Source: CAD feature listing. Evaluate the final solid. Frame: model axes, mm. Face numbers are marked on the shaded views. A direction names the side the tool comes from. Coordinates: 2 decimals unless noted, no trailing zeros. Order: outer loops, then holes, each group sorted by start corner. A loop starts at its lowest first (then second) coordinate and runs counter-clockwise, first axis right, second up. Notation, with made-up numbers: (47, -21.75) -> (61, -21.75) arc R9 ccw to (61, -8.75) -> close; hole circle Ø6 at (-30, 11.5). An arc over 180 degrees is marked (long way). Write item = value, one per line. Start each with the question number.
Item 1: Section query C-C (z = -56). Output: boundary loops of the cut face in (x, y), then the cut area to 3 significant figures.
Item 2: Mould query, pull axis X, two halves, no side actions, for the marked faces 1, 2 and 3. Classes: released by +X, released by -X, zero draft, split by the parting line, or undercut.
Item 3: Set-up query: the marked faces 4, 5, 6 and 7. Return all of +Z, -Z, +X, -X, +Y, -Y with unobstructed straight access to the full face (end or side cutting, diameter ignored); none if empty.
Item 4: Section query D-D (y = 31). Output: boundary loops of the cut face in (x, z), then the cut area to 3 significant figures.
Item 5: Ray query, line 1 along Z through (x, y) = (42.5, 44.5); line 2 along Z through (x, y) = (38, -8.5); line 3 along Z through (x, y) = (-79, 44.5). Return the intervals inside material, ascending. Write a range as [from, to].
Item 6: Section query B-B (y = 0). Output: boundary loops of the cut face in (x, z), then the cut area to 3 significant figures.
Item 7: Contact query for flat-ended pins moving along their axis: pin 1 (6 mm diameter, centred on y = -36.5, z = -48, fed in from -X); pin 2 (10 mm diameter, centred on x = 25.5, z = 32.5, fed in from -Y); pin 3 (6 mm diameter, centred on y = 2, z = 14, fed in from +X). Output: stop coordinate, or through.
Item 8: Section query A-A (x = 0). Output: boundary loops of the cut face in (y, z), then the cut area to 3 significant figures.
```python
from build123d import *

# Parameters (mm, degrees)
BOSS_EXTRUDE1_DEPTH = 200
BOSS_EXTRUDE2_DEPTH = 5
SKETCH3_R           = 37.5
BOSS_EXTRUDE3_DEPTH = 27
SKETCH4_R           = 37.5
BOSS_EXTRUDE4_DEPTH = 25
SKETCH5_R           = 45
BOSS_EXTRUDE5_DEPTH = 19


with BuildPart() as part:
    # Sketch1 → Boss-Extrude1 (new body)
    with BuildSketch(Plane.XY):
        Polygon((-127.5, 50), (-137.5, -50), (137.5, -50), (127.5, 50), align=None)
    extrude(amount=-BOSS_EXTRUDE1_DEPTH)

    # Sketch2 → Boss-Extrude2 (add)
    with BuildSketch(Plane(origin=(0, 0, 0), x_dir=(-1, 0, 0), z_dir=(0, 0, -1))):
        Polygon((-75, 50), (-65, -50), (65, -50), (75, 50), align=None)
    extrude(amount=-BOSS_EXTRUDE2_DEPTH)

    # Sketch3 → Boss-Extrude3 (add)
    with BuildSketch(Plane.XY.offset(5)):
        Circle(SKETCH3_R)
    extrude(amount=BOSS_EXTRUDE3_DEPTH)

    # Sketch4 → Boss-Extrude4 (add)
    with BuildSketch(Plane.XY.offset(32)):
        with BuildLine():
            ThreePointArc((-13.263603946, -35.076014745), (-37.5, 0), (-13.263603946, 35.076014745))
            Line((-13.263603946, 35.076014745), (-53.023534566, 50))
            Line((-53.023534566, 50), (-77.5, 36.492065403))
            Line((-77.5, 36.492065403), (-70.015632516, -50))
            Line((-70.015632516, -50), (-47.291260559, -50))
            Line((-47.291260559, -50), (-13.263603946, -35.076014745))
        make_face()
        Circle(SKETCH4_R)
        with BuildLine():
            Line((53.023534566, 50), (13.263603946, 35.076014745))
            ThreePointArc((13.263603946, 35.076014745), (30.851540869, 21.317420717), (37.5, 0))
            ThreePointArc((37.5, 0), (30.851540869, -21.317420717), (13.263603946, -35.076014745))
            Line((13.263603946, -35.076014745), (47.291260559, -50))
            Line((47.291260559, -50), (70.015632516, -50))
            Line((70.015632516, -50), (77.5, 36.492065403))
            Line((77.5, 36.492065403), (53.023534566, 50))
        make_face()
    extrude(amount=BOSS_EXTRUDE4_DEPTH)

    # Sketch5 → Boss-Extrude5 (add)
    with BuildSketch(Plane.XY.offset(57)):
        Circle(SKETCH5_R)
    extrude(amount=BOSS_EXTRUDE5_DEPTH)


solid = part.part
```
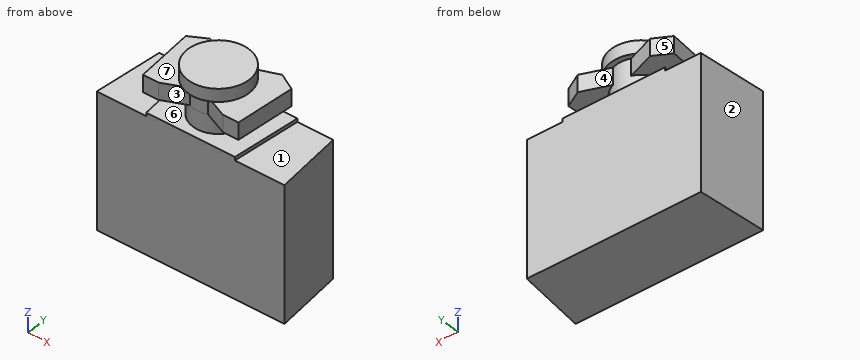
Computed:
q1.outline = (-137.5, -50) -> (137.5, -50) -> (127.5, 50) -> (-127.5, 50) -> close
q1.area = 26,500 mm^2
q2.face_1 = zero draft
q2.face_2 = released by -X
q2.face_3 = undercut
q3.face_4 = +Y
q3.face_5 = +Z, -X, +Y
q3.face_6 = none
q3.face_7 = +Z, -X
q4.outline = (-129.4, -200) -> (129.4, -200) -> (129.4, 0) -> (73.1, 0) -> (73.1, 5) -> (21.1, 5) -> (21.1, 32) -> (77.02, 32) -> (77.02, 57) -> (32.62, 57) -> (32.62, 76) -> (-32.62, 76) -> (-32.62, 57) -> (-77.02, 57) -> (-77.02, 32) -> (-21.1, 32) -> (-21.1, 5) -> (-73.1, 5) -> (-73.1, 0) -> (-129.4, 0) -> close
q4.area = 58,700 mm^2
q5.line_1 = [-200, 5], [32, 57]
q5.line_2 = [-200, 5], [32, 76]
q5.line_3 = [-200, 0]
q6.outline = (-132.5, -200) -> (132.5, -200) -> (132.5, 0) -> (70, 0) -> (70, 5) -> (37.5, 5) -> (37.5, 32) -> (74.34, 32) -> (74.34, 57) -> (45, 57) -> (45, 76) -> (-45, 76) -> (-45, 57) -> (-74.34, 57) -> (-74.34, 32) -> (-37.5, 32) -> (-37.5, 5) -> (-70, 5) -> (-70, 0) -> (-132.5, 0) -> close
q6.area = 61,200 mm^2
q7.pin_1 = -136.45
q7.pin_2 = -42.64
q7.pin_3 = 37.5
q8.outline = (-50, -200) -> (50, -200) -> (50, 5) -> (37.5, 5) -> (37.5, 57) -> (45, 57) -> (45, 76) -> (-45, 76) -> (-45, 57) -> (-37.5, 57) -> (-37.5, 5) -> (-50, 5) -> close
q8.area = 26,100 mm^2
